from build123d import *

# Parameters (mm, degrees)
SKETCH_W     = 14
SKETCH_H     = 14
PAD_DEPTH    = 5.9
POCKET_DEPTH = 55.319761


with BuildPart() as part:
    # Sketch → Pad (new body)
    with BuildSketch(Plane.XY):
        Rectangle(SKETCH_W, SKETCH_H)
    extrude(amount=PAD_DEPTH)

    # Sketch001 (on Face2 of Pad) → Pocket (cut, through all)
    with BuildSketch(Plane.YZ.offset(7)):
        Polygon((0, 6.9), (7, 6.9), (7, 5.9), (5.916667, 5.9), (5.916667, 1.4), (4.833333, 1.4), (4.833333, 5.9), (3.75, 5.9), (3.75, 1.4), (2.666667, 1.4), (2.666667, 5.9), (1.583333, 5.9), (1.583333, 1.4), (0.5, 1.4), (0.5, 5.9), (0, 5.9), align=None)
    pocket = extrude(amount=-POCKET_DEPTH, mode=Mode.SUBTRACT)

    # Mirrored: Pocket across XZ
    add(pocket.mirror(Plane.XZ), mode=Mode.SUBTRACT)


solid = part.part
Work out the finished part from the listing and answer in its coordinate system (mm). A direction names the side the tool comes from. Round coordinates to 2 decimals unless told otherwise and drop trailing zeros. Loops run counter-clockwise (first coordinate to the right, second up) from the corner with the lowest first, then second, coordinate; pieces in that order, holes last. Notation, with made-up numbers: M 29.25,17.5 L 68.25,17.5 A16 cw 68.25,32.5 Z; hole C 50.5,53.5 d3. An arc over 180 degrees is marked long. One line per question, with ' | ' between items. Start each with the question number.
(1) A tool of negligible diameter and unlimited length cuts with its end or side. For faces 4 (the face through (-0.1, 6.5, 5.9)), 5 (the face through (0, 2.667, 4)), from which of +Z, -Z, +X, -X, +Y, -Y can it reach the whole face along a straight path? Write none if from no direction.
(2) A flat-ended cylindrical pin translates along its axis: pin 1 Ø0.5 at (x, y) = (3, -1) entering from +Z. Find the tip coordinate at first contact, or state that the pin passes through.
(3) Find the intervals of material crossed by line 1 (Z direction, x = 0, y = 1.25), in increasing order.
(4) A cutting plane is placed at A-A on z = 5.25. Write down the section's boundary in (x, y), plus the area to 3 significant figures.
(5) A cutting plane is placed at C-C on y = -3. Write down the section's boundary in (x, z), plus the area to 3 significant figures.
(6) For a pull along Y with two mould halves and no side action, classify faces 1 (the face through (0, -4, 5.9)), 2 (the face through (0, -5, 1.4)), 3 (the face through (0, -0.5, 4)) as released by +Y, released by -Y, zero draft, split by the parting line, or undercut.
(7) A cutting plane is placed at B-B on x = 4.75. Write down the section's boundary in (y, z), plus the area to 4 significant figures.
Geometry check:
1) face 4: +Z, +X, -X, +Y, -Y | face 5: +Z, +X, -X
2) pin 1: stops at z = 1.4
3) line 1: z = 0 to 1.4
4) outline: M -7,-7 L 7,-7 L 7,-5.92 L -7,-5.92 Z; M -7,-4.83 L 7,-4.83 L 7,-3.75 L -7,-3.75 Z; M -7,-2.67 L 7,-2.67 L 7,-1.58 L -7,-1.58 Z; M -7,-0.5 L 7,-0.5 L 7,0.5 L -7,0.5 Z; M -7,1.58 L 7,1.58 L 7,2.67 L -7,2.67 Z; M -7,3.75 L 7,3.75 L 7,4.83 L -7,4.83 Z; M -7,5.92 L 7,5.92 L 7,7 L -7,7 Z | area: 105 mm²
5) outline: M -7,0 L 7,0 L 7,1.4 L -7,1.4 Z | area: 19.6 mm²
6) face 1: zero draft | face 2: undercut | face 3: undercut
7) outline: M -7,0 L 7,0 L 7,5.9 L 5.92,5.9 L 5.92,1.4 L 4.83,1.4 L 4.83,5.9 L 3.75,5.9 L 3.75,1.4 L 2.67,1.4 L 2.67,5.9 L 1.58,5.9 L 1.58,1.4 L 0.5,1.4 L 0.5,5.9 L -0.5,5.9 L -0.5,1.4 L -1.58,1.4 L -1.58,5.9 L -2.67,5.9 L -2.67,1.4 L -3.75,1.4 L -3.75,5.9 L -4.83,5.9 L -4.83,1.4 L -5.92,1.4 L -5.92,5.9 L -7,5.9 Z | area: 53.35 mm²
